Build history of the part. All positions in model axes, mm. A direction names the side the tool comes from. Round coordinates to 2 decimals unless told otherwise and drop trailing zeros. Write each loop counter-clockwise with the first axis right and the second up, starting at its lowest first coordinate (ties: lowest second). Pieces come first, ordered by that corner, then holes. Notation, with made-up numbers: (27.5, -25) -> (49.5, -25) arc R19 ccw to (49.5, 5) -> close; hole circle Ø4 at (-24, 6.25). An arc over 180 degrees is marked (long way). Return JSON: item names as keys, results as strings.
from build123d import *

# Parameters (mm, degrees)
SKETCH1_R           = 6.35
BOSS_EXTRUDE1_DEPTH = 1.984375
SKETCH2_R           = 6.35
BOSS_EXTRUDE2_DEPTH = 1.984375


with BuildPart() as part:
    # Sketch1 → Boss-Extrude1 (new body)
    with BuildSketch(Plane(origin=(0, 0, 0), x_dir=(1, 0, 0), z_dir=(0, 1, 0))):
        Polygon((0, 0), (34.925, 0), (34.925, -31.75), (31.75, -38.1), (3.175, -38.1), (0, -31.75), align=None)
        with Locations(Location((17.4625, -25.4, 0), (0, 0, 270))):
            Circle(SKETCH1_R, mode=Mode.SUBTRACT)
    extrude(amount=BOSS_EXTRUDE1_DEPTH)

    # Sketch2 → Boss-Extrude2 (add)
    with BuildSketch(Plane.XY):
        Polygon((0, 1.984375), (0, 46.434375), (3.175, 50.8), (31.75, 50.8), (34.925, 46.434375), (34.925, 1.984375), align=None)
        with Locations((17.4625, 38.1)):
            Circle(SKETCH2_R, mode=Mode.SUBTRACT)
    extrude(amount=BOSS_EXTRUDE2_DEPTH)


solid = part.part
Q1. 3-axis set-ups, long thin cutter, end or side, ignore diameter. For faces 5 (the flat face through (0, 16.2, 1.7)), 6 (the flat face through (18, 27, 1.984)): which of +Z, -Z, +X, -X, +Y, -Y reach the whole face in a straight line?
Verdict:
{"face 5": "+Z, -Z, -X, +Y, -Y", "face 6": "+Z, +X, -X, +Y"}
Q2. Saw through at D-D on x = 25.5. List the corners of the cut face in (y, z).
Verdict:
{"outline": "(0, 0) -> (50.8, 0) -> (50.8, 1.98) -> (1.98, 1.98) -> (1.98, 38.1) -> (0, 38.1) -> close"}
Q3. Pin check, flat tips, straight feed: pin 1 Ø10 at (x, y) = (17.46, 38.1) entering from +Z; pin 2 Ø17.5 at (x, y) = (22.5, 30) entering from +Z; pin 3 Ø16.5 at (x, z) = (17.46, 25.4) entering from +Y. Stop position of each tip, or through.
Verdict:
{"pin 1": "passes through", "pin 2": "stops at z = 1.98", "pin 3": "stops at y = 1.98"}
Q4. Saw through at A-A on y = 38.1. List the corners of the cut face in (x, z) (1 decimal).
Verdict:
{"outline": "(0, 0) -> (11.1, 0) -> (11.1, 2) -> (0, 2) -> close; (23.8, 0) -> (34.9, 0) -> (34.9, 2) -> (23.8, 2) -> close"}
Q5. Two-plate mould, pull along Z, no slides. Class faces 1 (the flat face through (1.61, 0.98, 34.97)), 2 (the cylindrical face through (21.754, 0.978, 20.72)), 3 (the flat face through (33.315, 48.648, 0.978)), 4 (the flat face through (18, 26, 0)): +Z half, -Z half, draft (parallel to the pull), parting line (faces both ways), or undercut.
Verdict:
{"face 1": "+Z half", "face 2": "undercut", "face 3": "draft", "face 4": "-Z half"}
Q6. Saw through at B-B on x = 13. List the corners of the cut face in (y, z), then the cut area to 3 significant figures.
Verdict:
{"outline": "(0, 0) -> (33.58, 0) -> (33.58, 1.98) -> (1.98, 1.98) -> (1.98, 20.88) -> (0, 20.88) -> close; (0, 29.92) -> (1.98, 29.92) -> (1.98, 38.1) -> (0, 38.1) -> close; (42.62, 0) -> (50.8, 0) -> (50.8, 1.98) -> (42.62, 1.98) -> close", "area": "137 mm²"}
Q7. Wall check: L1, parallel to X at y = 0.6, z = 25.4 (1 decimal); L2, parallel to Z at x = 31, y = 41. Give the ranges that are in metal, low to high.
Verdict:
{"L1": "x = 0 to 11.1, 23.8 to 34.9", "L2": "z = 0 to 1.98"}
